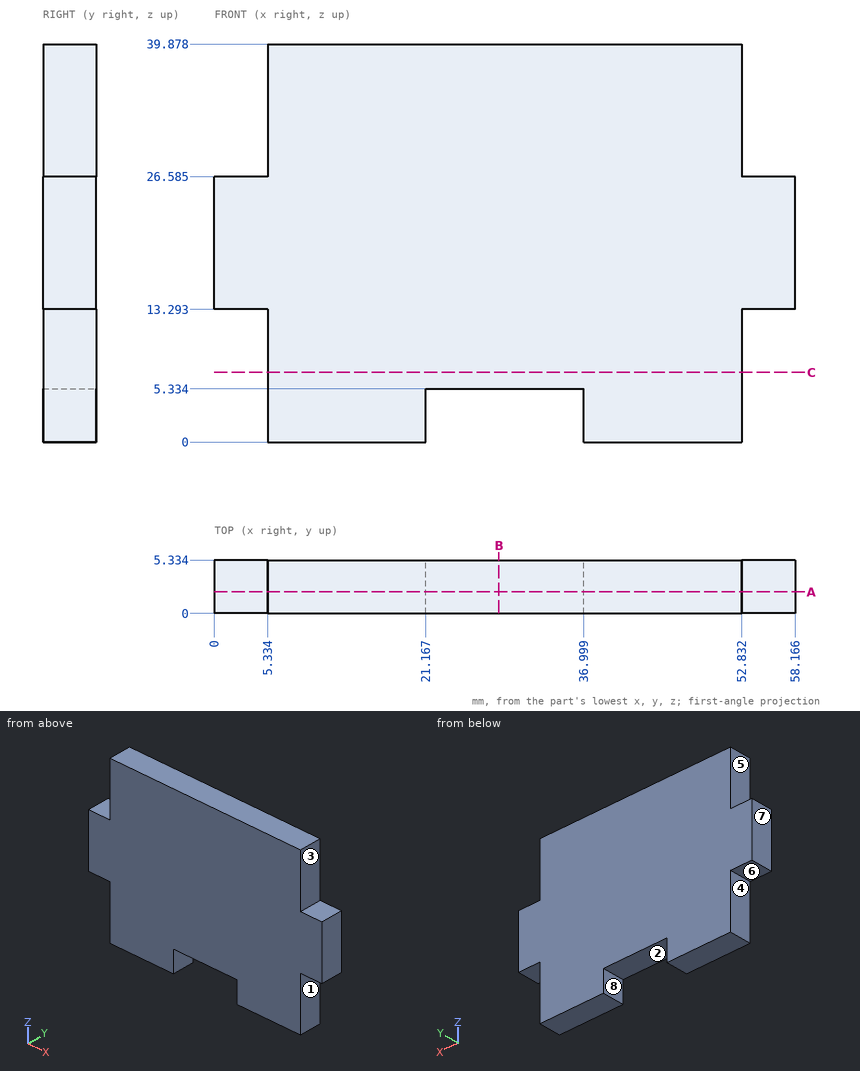
Verification items for this drawing (mm, ordinates from the low corner). A direction names the side the tool comes from. Round coordinates to 2 decimals unless told otherwise and drop trailing zeros. Order: outer loops, then holes, each group sorted by start corner. A loop starts at its lowest first (then second) coordinate and runs counter-clockwise, first axis right, second up. Notation, with made-up numbers: (72, 36.5) -> (86, 36.5) arc R25 ccw to (86, 64.5) -> close; hole circle Ø1 at (87.25, -10.5). An arc over 180 degrees is marked (long way). Use one line per item in the form item = value.
1. Scan lines: line 1 along X through (y, z) = (4.9, 2.5); line 2 along Z through (x, y) = (23.5, 4.2); line 3 along X through (y, z) = (1.1, 29.5). Record each from-to range of solid material in increasing order. Write a range as from..to.
Working result:
line_1 = 5.33..21.17, 37..52.83
line_2 = 5.33..39.88
line_3 = 5.33..52.83
2. Cross-section at A-A, the plane y = 2.15. Enter the section's corners in (x, z) (1 decimal), plus the area to 3 significant figures.
Working result:
outline = (0, 13.3) -> (5.3, 13.3) -> (5.3, 0) -> (21.2, 0) -> (21.2, 5.3) -> (37, 5.3) -> (37, 0) -> (52.8, 0) -> (52.8, 13.3) -> (58.2, 13.3) -> (58.2, 26.6) -> (52.8, 26.6) -> (52.8, 39.9) -> (5.3, 39.9) -> (5.3, 26.6) -> (0, 26.6) -> close
area = 1,950 mm^2
3. Cross-section at B-B, the plane x = 28.5. Enter the section's corners in (y, z).
Working result:
outline = (0, 5.33) -> (5.33, 5.33) -> (5.33, 39.88) -> (0, 39.88) -> close
4. Go/stop test with flat-tipped pins: pin 1 (2.5 mm diameter, centred on x = 55, y = 4, fed in from -Z); pin 2 (1.6 mm diameter, centred on x = 27, y = 2.5, fed in from -Z); pin 3 (1 mm diameter, centred on y = 0.5, z = 12.5, fed in from +X). Record where each tip stops, or that it passes through.
Working result:
pin_1 = 13.29
pin_2 = 5.33
pin_3 = 52.83
5. Mould release check, pull along X, two halves, no side actions. Record for the marked faces 6, 7 and 8: pulls with the +X half, pulls with the -X half, needs draft (parallel to the pull), parting line crosses it, or undercut.
Working result:
face_6 = needs draft
face_7 = pulls with the -X half
face_8 = undercut
6. Set-up check for the marked faces 1, 2, 3, 4 and 5: record each of +Z, -Z, +X, -X, +Y, -Y from which the full face is reachable in a straight line by a thin tool's end or side.
Working result:
face_1 = -Z, +X, +Y, -Y
face_2 = -Z, +Y, -Y
face_3 = +Z, +X, +Y, -Y
face_4 = -Z, -X, +Y, -Y
face_5 = +Z, -X, +Y, -Y
7. Cross-section at C-C, the plane z = 7. Enter the section's corners in (x, y), plus the area to 3 significant figures.
Working result:
outline = (5.33, 0) -> (52.83, 0) -> (52.83, 5.33) -> (5.33, 5.33) -> close
area = 253 mm^2
